from build123d import *

# Parameters (mm, degrees)
SKETCH1_W           = 900
SKETCH1_H           = 100
BOSS_EXTRUDE1_DEPTH = 20
SKETCH2_R           = 9.7
SKETCH2_R_2         = 4.826
BOSS_EXTRUDE2_DEPTH = 15.8


with BuildPart() as part:
    # Sketch1 → Boss-Extrude1 (new body)
    with BuildSketch(Plane.XY):
        Rectangle(SKETCH1_W, SKETCH1_H)
    extrude(amount=BOSS_EXTRUDE1_DEPTH)

    # Sketch2 → Boss-Extrude2 (add)
    # profile 1 of 3: a face of its own
    with BuildSketch(Plane.XY):
        with Locations((-300, -30.95)):
            Circle(SKETCH2_R)
        with Locations((-300, -30.95)):
            Circle(SKETCH2_R_2, mode=Mode.SUBTRACT)
    # profile 2 of 3: a face of its own
    with BuildSketch(Plane.XY):
        with Locations((0, -30.95)):
            Circle(SKETCH2_R)
        with Locations((0, -30.95)):
            Circle(SKETCH2_R_2, mode=Mode.SUBTRACT)
    # profile 3 of 3: a face of its own
    with BuildSketch(Plane.XY):
        with Locations((300, -30.95)):
            Circle(SKETCH2_R)
        with Locations((300, -30.95)):
            Circle(SKETCH2_R_2, mode=Mode.SUBTRACT)
    extrude(amount=-BOSS_EXTRUDE2_DEPTH)


solid = part.part
Input: part model. Units: mm. Frame: model coordinates. A direction names the side the tool comes from. Give positions to 0.01 mm unless a question says otherwise; leave off trailing zeros. Order: outer loops, then holes, each group sorted by start corner. A loop starts at its lowest first (then second) coordinate and runs counter-clockwise, first axis right, second up.
Q1. Draft query along X for faces 3 (the flat face through (-6, 1, 20)), 4 (the flat face through (-6, 1, 0)), 5 (the cylindrical face through (-290.748, -28.036, -7.789)), 6 (the flat face through (450, -1, 10)). Return one class per face: +X half, -X half, draft (parallel to the pull), parting line (faces both ways), or undercut.
Checked values:
face 3: draft
face 4: undercut
face 5: undercut
face 6: +X half
Q2. Section B-B on y = 17.5. Output: boundary loops of the cut face in (x, z).
Checked values:
outline: (-450, 0) - (450, 0) - (450, 20) - (-450, 20) - close
Q3. Section A-A on x = 172. Output: boundary loops of the cut face in (y, z).
Checked values:
outline: (-50, 0) - (50, 0) - (50, 20) - (-50, 20) - close
Q4. Set-up query: faces 1 (the flat face through (-2.3, -26.5, -15.8)), 2 (the cylindrical face through (-1.263, -21.333, -7.789)). Return all of +Z, -Z, +X, -X, +Y, -Y with unobstructed straight access to the full face (end or side cutting, diameter ignored); none if empty.
Checked values:
face 1: -Z, +X, -X, +Y, -Y
face 2: -Z
Q5. Ray query, probe 1 along X at (y, z) = (-30, -4); probe 2 along Y at (x, z) = (0, -11.75); probe 3 along X at (y, z) = (-39.5, -2). Return the intervals inside material, ascending.
Checked values:
probe 1: x = -309.65 to -304.73, -295.27 to -290.35, -9.65 to -4.73, 4.73 to 9.65, 290.35 to 295.27, 304.73 to 309.65
probe 2: y = -40.65 to -35.78, -26.12 to -21.25
probe 3: x = -304.58 to -295.42, -4.58 to 4.58, 295.42 to 304.58
Q6. Contact query for flat-ended pins moving along their axis: pin 1 Ø6 at (y, z) = (-26.5, -8.5) entering from -X; pin 2 Ø5 at (x, y) = (169, -16.5) entering from -Z. Output: stop coordinate, or through.
Checked values:
pin 1: stops at x = -309.59
pin 2: stops at z = 0
